Read the model definition and answer for the solid it produces. Units are mm, in the model's axes. A direction names the side the tool comes from. Coordinates: 2 decimals unless noted, no trailing zeros. Loops run counter-clockwise (first coordinate to the right, second up) from the corner with the lowest first, then second, coordinate; pieces in that order, holes last.
Q1. Section A-A (z = -1.25) is taken. Give the vertices of the cut face in (x, y) (3 decimals), then the cut area to 3 significant figures.
Q2. Flat-ended cylindrical pins translate along their axes: P1, Ø1.5, axis at y = 69.5, z = -2, coming from the +X side; P2, Ø1.5, axis at x = -37.5, z = -4, coming from the +Y side (3 decimals); P3, Ø1, axis at y = 65.5, z = -2.5, coming from the +X side. Find the tip coordinate at first contact, or state that the pin passes through.
Q3. Which of the six approach directions +Z, -Z, +X, -X, +Y, -Y give full straight-line access (tool end or side, diameter ignored) to faces 1 (the face through (-35.945, 64.21, -2.317)), 2 (the face through (-38, 67, 1)), 3 (the face through (-34.39, 66.72, 0))?
Q4. Straight lines are drawn through the part: line 1 (Y direction, x = -38, z = -3) (3 decimals); line 2 (X direction, y = 70, z = -0.75); line 3 (X direction, y = 68, z = -2.5). For each, find the intervals that lie inside material, in ascending order.
Q5. Section B-B (x = -38) is taken. Give the vertices of the cut face in (y, z) (3 decimals), then the cut area to 3 significant figures.
from build123d import *

# Parameters (mm, degrees)
ESQUISSE1_R                  = 3.465
BOSS_EXTRU_1_DEPTH           = 5
ESQUISSE2_R                  = 4.15
BOSS_EXTRU_2_DEPTH           = 1
CONG_1_R                     = 0.5
BOSS_EXTRU_3_DEPTH           = 9
BOSS_EXTRU_3_DEPTH_BACK      = 2
ENL_V_START                  = -4
ENL_V_MAT_EXTRU_1_DEPTH      = 4
CHANFREIN1_SIZE              = 0.3
ENL_V_MAT_EXTRU_2_REACH      = 84.915
ENL_V_MAT_EXTRU_2_END_RADIUS = 8


with BuildPart() as part:
    # Esquisse1 → Boss.-Extru.1 (new body)
    with BuildSketch(Plane.XY):
        with Locations((-38, 67)):
            Circle(ESQUISSE1_R)
    extrude(amount=-BOSS_EXTRU_1_DEPTH)

    # Esquisse2 → Boss.-Extru.2 (add)
    with BuildSketch(Plane.XY):
        with Locations((-38, 67)):
            Circle(ESQUISSE2_R)
    extrude(amount=BOSS_EXTRU_2_DEPTH)

    # Congé1
    cong_1_edges = [part.edges().sort_by_distance(p)[0] for p in [
        (-42.15, 67, 1),
    ]]
    fillet(cong_1_edges, radius=CONG_1_R)

    # Esquisse4 → Boss.-Extru.3 (add, two sides: drawn at the far end of the back side and taken through both)
    with BuildSketch(Plane(origin=(29.785, 71.15, 0), x_dir=(0, 0, 1), z_dir=(0, -1, 0)).offset(-BOSS_EXTRU_3_DEPTH_BACK)):
        with BuildLine():
            Line((0, 71.935), (-1.84883954, 71.935))
            ThreePointArc((-1.84883954, 71.935), (-0.476394359, 69.539440781), (0, 66.82))
            Line((0, 66.82), (0, 71.935))
        make_face()
    extrude(amount=BOSS_EXTRU_3_DEPTH + BOSS_EXTRU_3_DEPTH_BACK)

    # Esquisse5 → Enlèv. mat.-Extru.1 (cut)
    with BuildSketch(Plane.XY.offset(1).offset(ENL_V_START)):
        with BuildLine():
            Line((-37.035, 62.963754839), (-36.628505561, 58.672971398))
            Line((-36.628505561, 58.672971398), (-43.808246532, 59.466119951))
            Line((-43.808246532, 59.466119951), (-42.997006725, 73.486489438))
            Line((-42.997006725, 73.486489438), (-36.628505561, 73.524507843))
            Line((-36.628505561, 73.524507843), (-37.035, 71.036245161))
            ThreePointArc((-37.035, 71.036245161), (-40.57077323, 70.25785589), (-42.15, 67))
            ThreePointArc((-42.15, 67), (-40.57077323, 63.74214411), (-37.035, 62.963754839))
        make_face()
    extrude(amount=ENL_V_MAT_EXTRU_1_DEPTH, mode=Mode.SUBTRACT)

    # Chanfrein1
    chanfrein1_edges = [part.edges().sort_by_distance(p)[0] for p in [
        (-41.465, 67, -5),
    ]]
    chamfer(chanfrein1_edges, length=CHANFREIN1_SIZE)

    # Enlèv. mat.-Extru.2: up to this cylinder (the profile starts inside it)
    enl_v_mat_extru_2_end = Plane(origin=(-37.035, 70.315316, -8), z_dir=(0, -1, 0)) * Cylinder(ENL_V_MAT_EXTRU_2_END_RADIUS, 186.83, mode=Mode.PRIVATE)
    # Esquisse7 → Enlèv. mat.-Extru.2 (cut, up to the surface)
    with BuildSketch(Plane(origin=(0, 0, -5), x_dir=(-1, 0, 0), z_dir=(0, 0, -1)), mode=Mode.PRIVATE) as enl_v_mat_extru_2_sk1:
        with BuildLine():
            Line((36.707715202, 70.215), (39.292284798, 70.215))
            ThreePointArc((39.292284798, 70.215), (38.173107277, 70.460673182), (37.035, 70.327912258))
            ThreePointArc((37.035, 70.327912258), (36.869946479, 70.275546373), (36.707715202, 70.215))
        make_face()
    enl_v_mat_extru_2_tool1 = extrude(enl_v_mat_extru_2_sk1.sketch, amount=-ENL_V_MAT_EXTRU_2_REACH, mode=Mode.PRIVATE) & enl_v_mat_extru_2_end
    add(enl_v_mat_extru_2_tool1.solids().sort_by_distance((-38, 70.315316, -5))[0], mode=Mode.SUBTRACT)


solid = part.part
Numbers:
1. outline: (-41.329, 64.522) - (-41.329, 66.038) arc R3.465 ccw (long way) to (-36.708, 70.215) - (-39.292, 70.215) arc R3.465 ccw to (-41.329, 67.962) - (-41.329, 69.478) arc R4.15 ccw to start
1. area: 39.9 mm2
2. P1: stops at x = -35.01
2. P2: stops at y = 70.215
2. P3: stops at x = -34.68
3. face 1: -Z
3. face 2: +Z, +X, -X, +Y, -Y
3. face 3: -Z, +X
4. line 1: y = 63.535 to 70.215
4. line 2: x = -40.87 to -40.42, -39.73 to -36.27
4. line 3: x = -41.32 to -34.68
5. outline: (62.85, -0.058) - (63.535, -0.058) - (63.535, -4.7) - (63.835, -5) - (70.165, -5) - (70.215, -4.95) - (70.215, -0.058) - (71.15, -0.058) - (71.15, 0.5) arc R0.5 ccw to (70.65, 1) - (63.35, 1) arc R0.5 ccw to (62.85, 0.5) - close
5. area: 41.6 mm2
